Part model, mm, in its own coordinate system. A direction names the side the tool comes from. Coordinates: 2 decimals unless noted, no trailing zeros. Loops run counter-clockwise (first coordinate to the right, second up) from the corner with the lowest first, then second, coordinate; pieces in that order, holes last. Notation, with made-up numbers: M 53.5,-34 L 112.5,-34 A20 ccw 112.5,-11 Z; hole C 70.25,4 d5. An arc over 180 degrees is marked long. Answer as a JSON object with one key per item and string values. Group by question number.
1. Drill centre lines: L1, parallel to X at y = -4.5, z = 4.5; L2, parallel to X at y = -8, z = 13.5; L3, parallel to X at y = -7, z = 8. Where is each one in solid material? Low to high.
2. Mould opens along X. For faces 4 (the face through (-13.039, -7.605, 7.395)), 5 (the face through (-57, -29.82, 7)), 6 (the face through (-61.489, -2, 7)) say: released by +X, released by -X, zero draft, split by the parting line, or undercut.
3. Saw through at A-A on x = 140.5. Write the cut outline in (y, z), then the cut area to 3 significant figures.
4. Saw through at D-D on x = 9. Write the cut outline in (y, z).
5. Drop flat-ended pins along their axis: pin 1 Ø1 at (y, z) = (21.5, 3.5) entering from +X; pin 2 Ø1 at (y, z) = (-6, 4) entering from +X; pin 3 Ø3 at (x, z) = (64, 4) entering from +Y. Give the stop position or say it passes through.
6. Saw through at B-B on y = 15. Write the cut outline in (x, z).
7. Saw through at C-C on z = 4.25. Write the cut outline in (x, y).
8. 3-axis set-ups, long thin cutter, end or side, ignore diameter. For faces 1 (the face through (73, 9, 15)), 2 (the face through (-41.489, -8, 7)), 3 (the face through (17, 25, 7)): which of +Z, -Z, +X, -X, +Y, -Y reach the whole face in a straight line?
from build123d import *

# Parameters (mm, degrees)
F0_R     = 17.5
F0_W     = 10
F0_H     = 0.180238
F0_H_2   = 29.819762
F0_W_2   = 8
F0_H_3   = 15
F1_DEPTH = 15


with BuildPart() as f1:
    # F0 (on Top) → F1 (new body)
    with BuildSketch(Plane.XY):
        with BuildLine():
            Line((93.510551, 25), (-61.489449, 25))
            Line((-61.489449, 25), (-61.489449, 0.180238))
            Line((-61.489449, 0.180238), (-51.489449, 0.180238))
            Line((-51.489449, 0.180238), (-51.489449, 0))
            Line((-51.489449, 0), (-41.489449, 0))
            Line((-41.489449, 0), (-33.489449, 0))
            Line((-33.489449, 0), (-23.489449, 0))
            Line((-23.489449, 0), (-9.489449, 0))
            Line((-9.489449, 0), (92.862259, 0))
            ThreePointArc((92.862259, 0), (160.853792, 10.745271), (93.510551, 25))
        make_face()
        with Locations((125.865554, 11.652575)):
            Circle(F0_R, mode=Mode.SUBTRACT)
        with Locations((-56.489449, 0.090119)):
            Rectangle(F0_W, F0_H)
        with Locations((-56.489449, -14.909881)):
            Rectangle(F0_W, F0_H_2)
        Polygon((-16.489578, -15), (-9.489449, 0), (-23.489449, 0), align=None)
        with Locations((-37.489449, -7.5)):
            Rectangle(F0_W_2, F0_H_3)
    extrude(amount=F1_DEPTH)


solid = f1.part
Outcome:
{
 "1": {"L1": "x = -61.49 to -51.49, -41.49 to -33.49, -21.39 to -11.59, 94.82 to 119.13, 132.6 to 156.92", "L2": "x = -61.49 to -51.49, -41.49 to -33.49, -19.76 to -13.22, 96.9 to 154.83", "L3": "x = -61.49 to -51.49, -41.49 to -33.49, -20.22 to -12.76, 96.25 to 155.48"},
 "2": {"face 4": "undercut", "face 5": "zero draft", "face 6": "released by -X"},
 "3": {"outline": "M -20.14,0 L 2.06,0 L 2.06,15 L -20.14,15 Z; M 21.25,0 L 43.45,0 L 43.45,15 L 21.25,15 Z", "area": "666 mm²"},
 "4": {"outline": "M 0,0 L 25,0 L 25,15 L 0,15 Z"},
 "5": {"pin 1": "stops at x = 159.59", "pin 2": "stops at x = 156.37", "pin 3": "stops at y = 25"},
 "6": {"outline": "M -61.49,0 L 108.69,0 L 108.69,15 L -61.49,15 Z; M 143.04,0 L 160.71,0 L 160.71,15 L 143.04,15 Z"},
 "7": {"outline": "M -61.49,-29.82 L -51.49,-29.82 L -51.49,0 L -41.49,0 L -41.49,-15 L -33.49,-15 L -33.49,0 L -23.49,0 L -16.49,-15 L -9.49,0 L 92.86,0 A35 ccw long 93.51,25 L -61.49,25 Z; hole C 125.87,11.65 d35"},
 "8": {"face 1": "+Z, +X, -X, +Y, -Y", "face 2": "+Z, -Z, -Y", "face 3": "+Z, -Z, -X, +Y"}
}
